from build123d import *

# Parameters (mm, degrees)
F0_R     = 8
F1_DEPTH = 1.25
F2_R     = 1.05
F3_DEPTH = 25
F4_R     = 1.05
F5_DEPTH = 0.75


with BuildPart() as f1:
    # F0 (on Top) → F1 (new body)
    with BuildSketch(Plane.XY):
        Circle(F0_R)
    extrude(amount=F1_DEPTH)

    # F2 (on face) → F3 (cut)
    with BuildSketch(Plane.XY.offset(1.25)):
        Circle(F2_R)
    extrude(amount=-F3_DEPTH, mode=Mode.SUBTRACT)

    # F4 (on face) → F5 (cut)
    with BuildSketch(Plane.XY.offset(1.25)):
        with Locations((0, 6.25)):
            Circle(F4_R)
        with Locations((-4.419417, 4.419417)):
            Circle(F4_R)
        with Locations((-6.25, 0)):
            Circle(F4_R)
        with Locations((-4.419417, -4.419417)):
            Circle(F4_R)
        with Locations((0, -6.25)):
            Circle(F4_R)
        with Locations((4.419417, -4.419417)):
            Circle(F4_R)
        with Locations((6.25, 0)):
            Circle(F4_R)
        with Locations((4.419417, 4.419417)):
            Circle(F4_R)
    extrude(amount=-F5_DEPTH, mode=Mode.SUBTRACT)


solid = f1.part
Geometry: final body of the model. Coordinates: model frame, mm. A direction names the side the tool comes from. Coordinates: 2 decimals unless noted, no trailing zeros. Order: outer loops, then holes, each group sorted by start corner. A loop starts at its lowest first (then second) coordinate and runs counter-clockwise, first axis right, second up. Notation, with made-up numbers: M -22.5,35.5 L -4.5,35.5 A14 ccw -4.5,56.5 Z; hole C -13,-11.75 d7. An arc over 180 degrees is marked long. One line per question, with ' | ' between items. Start each with the question number.
Item 1: Cut plane C-C, the plane z = 0.7. Count the separate pieces of the cut face and the enclosed holes in it, then the cut area to 3 significant figures.
Item 2: Set-up query: faces 4 (the flat face through (-6, 0, 0.5)), 5 (the flat face through (0, -2, 1.25)). Return all of +Z, -Z, +X, -X, +Y, -Y with unobstructed straight access to the full face (end or side cutting, diameter ignored); none if empty.
Item 3: Cut plane A-A, the plane x = 0. Return the cut outline in (y, z).
Item 4: Cut plane D-D, the plane y = -6.25. Return the cut outline in (x, z), then the cut area to 3 significant figures.
Item 5: Ray query, probe 1 along Y at (x, z) = (0, 0.8); probe 2 along Y at (x, z) = (5, 0.95) (3 decimals); probe 3 along X at (y, z) = (-0.75, 1.1). Return the intervals inside material, ascending. Write a range as [from, to].
Item 6: Draft query along X for faces 1 (the cylindrical face through (-0.14, -5.21, 0.88)), 2 (the cylindrical face through (-1.73, -7.81, 0.62)), 3 (the flat face through (2, 0, 0)). Return one class per face: released by +X, released by -X, zero draft, split by the parting line, or undercut.
Item 7: Pin query (flat end, axial travel): pin 1 Ø1.3 at (x, y) = (0, 6.25) entering from +Z; pin 2 Ø1.5 at (x, y) = (6.5, 1) entering from -Z. Return the tip coordinate at first contact, or that it passes through.
A:
1) separate pieces: 1 | enclosed holes: 9 | area: 170 mm2
2) face 4: +Z | face 5: +Z, +X, -X, +Y, -Y
3) outline: M -8,0 L -1.05,0 L -1.05,1.25 L -5.2,1.25 L -5.2,0.5 L -7.3,0.5 L -7.3,1.25 L -8,1.25 Z; M 1.05,0 L 8,0 L 8,1.25 L 7.3,1.25 L 7.3,0.5 L 5.2,0.5 L 5.2,1.25 L 1.05,1.25 Z
4) outline: M -4.99,0 L 4.99,0 L 4.99,1.25 L 1.05,1.25 L 1.05,0.5 L -1.05,0.5 L -1.05,1.25 L -4.99,1.25 Z | area: 10.9 mm2
5) probe 1: y = [-8, -7.3], [-5.2, -1.05], [1.05, 5.2], [7.3, 8] | probe 2: y = [-6.245, -5.294], [-3.545, 3.545], [5.294, 6.245] | probe 3: x = [-7.96, -6.98], [-5.52, -0.73], [0.73, 5.52], [6.98, 7.96]
6) face 1: undercut | face 2: split by the parting line | face 3: zero draft
7) pin 1: stops at z = 0.5 | pin 2: stops at z = 0
